Check sheet for the modelled part. Datum: model origin and axes. Units: mm. A direction names the side the tool comes from. Coordinates: 2 decimals unless noted, no trailing zeros. Order: outer loops, then holes, each group sorted by start corner. A loop starts at its lowest first (then second) coordinate and runs counter-clockwise, first axis right, second up.
1. Cross-section at A-A (x = 20). Enter the section's corners in (y, z), then the cut area to 3 significant figures.
2. Thickness scan on line 1 (Y direction, x = -5, z = -9.75); line 2 (Y direction, x = 11, z = -4). Record the ranges inside material, lowest first.
3. Set-up check for faces 1 (the flat face through (25, 0, 0)), 2 (the cylindrical face through (18.53, -0.54, -2.44)): record each of +Z, -Z, +X, -X, +Y, -Y from which the full face is reachable in a straight line by a thin tool's end or side.
4. Gauge pin test, flat ends, axial feed: pin 1 Ø8 at (x, y) = (9, -8.5) entering from +Z; pin 2 Ø2 at (x, z) = (-1, -2) entering from +Y; pin 3 Ø8 at (x, z) = (18.5, 1) entering from +Y. Record the tip position at first contact, or that the pin passes through.
```python
from build123d import *

# Parameters (mm, degrees)
F0_R     = 12.5
F1_DEPTH = 12.5
F2_R     = 12.49999
F3_R     = 2.5
F4_DEPTH = 25


# Not quite as in the source:
# - a fillet or chamfer is up to 0.001 mm smaller than in the source, because OpenCascade refuses the exact size


with BuildPart() as f1:
    # F0 (on Front) → F1 (new body, symmetric)
    with BuildSketch(Plane.XZ):
        Circle(F0_R)
    extrude(amount=F1_DEPTH, both=True)

    # F2 (radius 12.5 in the source; OpenCascade refuses exactly that, so slightly less here)
    f2_edges = [f1.edges().sort_by_distance(p)[0] for p in [
        (-12.5, -12.5, 0),
        (-12.5, 12.5, 0),
    ]]
    fillet(f2_edges, radius=F2_R)

    # F3 (on Right) → F4 (join)
    with BuildSketch(Plane.YZ):
        Circle(F3_R)
    extrude(amount=F4_DEPTH)


solid = f1.part
```
Data:
1. outline: circle Ø5 at (0, 0)
1. area: 19.6 mm2
2. line 1: y = -6.02 to 6.02
2. line 2: y = -4.39 to 4.39
3. face 1: +Z, -Z, +X, +Y, -Y
3. face 2: +X
4. pin 1: stops at z = 9.28
4. pin 2: stops at y = 12.44
4. pin 3: stops at y = 2.5
